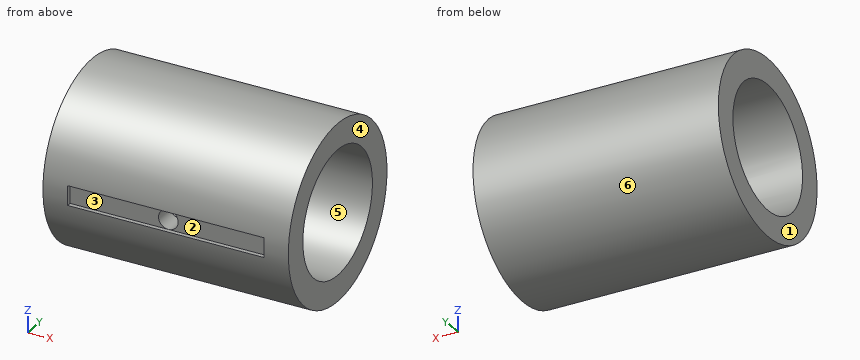
Solid Edge part; units mm, degrees
sketch "Sketch1" plane through (0, 0, 0) normal (1, 0, 0) x (0, 1, 0)
  circle A0 centre (0, 0) radius 9
  circle A1 centre (0, 0) radius 6.35
extrude "Protrusion1" add sketch "Sketch1" along normal mid plane 25
sketch "Sketch2" plane through (0, -9, 0) normal (0, -1, 0) x (1, 0, 0)
  line L0 (10, -1) -> (-10, -1)
  line L1 (-10, -1) -> (-10, 1)
  line L2 (-10, 1) -> (10, 1)
  line L3 (10, 1) -> (10, -1)
extrude "ExtrudedCutout_1" cut sketch "Sketch2" against normal blind 0.5
hole "Hole_1" at (0, -9, 0) direction (0, 1, 0) diameter 2 end up to next
For this review, take the finished solid that the model builds, in its own axes (mm). Face numbers are marked on the shaded views. A direction names the side the tool comes from. Give positions to 0.01 mm unless a question says otherwise; leave off trailing zeros. Write each loop counter-clockwise with the first axis right and the second up, starting at its lowest first coordinate (ties: lowest second). Pieces come first, ordered by that corner, then holes. Notation, with made-up numbers: M -37.5,-21.5 L -9.5,-21.5 A9 ccw -9.5,-7.5 Z; hole C 58,40 d10. An arc over 180 degrees is marked long. Answer as a JSON object with one key per item and string values. Group by question number.
Item 1: Tool access review of the marked faces 1 and 2: name each direction out of +Z, -Z, +X, -X, +Y, -Y from which nothing blocks a thin tool from reaching the whole face with its end or side.
Item 2: Consider section C-C on x = 7.25. Write out the cut boundary in (y, z), plus the area to 3 significant figures.
Item 3: Consider section A-A on y = 0. Write out the cut boundary in (x, z), plus the area to 4 significant figures.
Item 4: Consider section D-D on z = 2.5. Write out the cut boundary in (x, y), plus the area to 3 significant figures.
Item 5: For pin 1 Ø8 at (x, z) = (-2.5, 4.5) entering from -Y; pin 2 Ø1.5 at (x, z) = (7, -1) entering from +Y; pin 3 Ø6 at (x, y) = (-0.5, 2) entering from -Z; pin 4 Ø1 at (x, y) = (-7.5, 1.5) entering from +Z, all flat-tipped, find the tip position at first contact; note any pin that passes through.
Item 6: For probe 1 along Y at (x, z) = (7, 0); probe 2 along Z at (x, y) = (-0.75, 0); probe 3 along Z at (x, y) = (4.5, -1), list the stretches that pass through material, from the lowest coordinate up. Write a range as [from, to].
Item 7: Draft analysis for pull direction Z (two halves, no side actions). For the marked faces 3, 4, 5 and 6, state which applies: +Z half, -Z half, draft (parallel to the pull), parting line (faces both ways), or undercut.
Item 8: Consider section B-B on z = 0. Write out the cut boundary in (x, y).
Check result:
{
 "1": {"face 1": "+Z, -Z, -X, +Y, -Y", "face 2": "-Y"},
 "2": {"outline": "M -8.94,-1 A9 ccw long -8.94,1 L -8.5,1 L -8.5,-1 Z; hole C 0,0 d12.7", "area": "127 mm^2"},
 "3": {"outline": "M -12.5,-9 L 12.5,-9 L 12.5,-6.35 L -12.5,-6.35 Z; M -12.5,6.35 L 12.5,6.35 L 12.5,9 L -12.5,9 Z", "area": "132.5 mm^2"},
 "4": {"outline": "M -12.5,-8.65 L 12.5,-8.65 L 12.5,-5.84 L -12.5,-5.84 Z; M -12.5,5.84 L 12.5,5.84 L 12.5,8.65 L -12.5,8.65 Z", "area": "140 mm^2"},
 "5": {"pin 1": "stops at y = -8.94", "pin 2": "stops at y = 9", "pin 3": "stops at z = -9", "pin 4": "stops at z = 8.94"},
 "6": {"probe 1": "y = [-8.5, -6.35], [6.35, 9]", "probe 2": "z = [-9, -6.35], [6.35, 9]", "probe 3": "z = [-8.94, -6.27], [6.27, 8.94]"},
 "7": {"face 3": "undercut", "face 4": "draft", "face 5": "undercut", "face 6": "parting line"},
 "8": {"outline": "M -12.5,-9 L -10,-9 L -10,-8.5 L -1,-8.5 L -1,-6.35 L -12.5,-6.35 Z; M -12.5,6.35 L 12.5,6.35 L 12.5,9 L -12.5,9 Z; M 1,-8.5 L 10,-8.5 L 10,-9 L 12.5,-9 L 12.5,-6.35 L 1,-6.35 Z"}
}
